Could you check a few things on this model? Use its own coordinates, in mm. Face numbers are marked on the shaded views. Round coordinates to 2 decimals unless told otherwise and drop trailing zeros. Loops run counter-clockwise (first coordinate to the right, second up) from the corner with the lowest first, then second, coordinate; pieces in that order, holes last. Notation, with made-up numbers: M 5.5,70.5 L 23.5,70.5 A13 cw 23.5,77.5 Z; hole C 68.5,58.25 d5. An arc over 180 degrees is marked long. Answer in a Markdown table with one row per item.
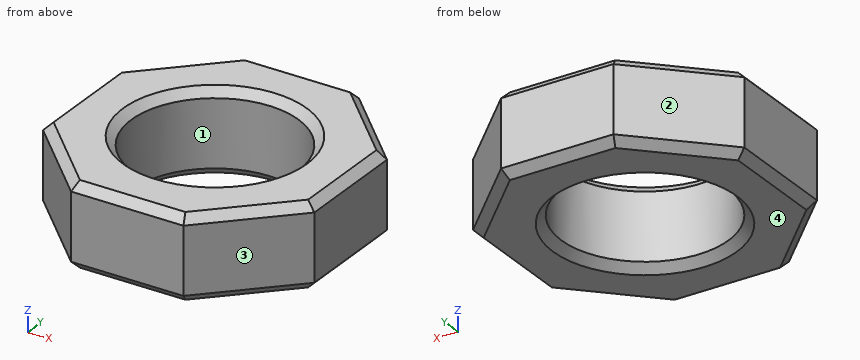
```python
from build123d import *

# Parameters (mm, degrees)
F1_DEPTH = 20
F2_R     = 20
F3_DEPTH = 20.001
F4_SIZE  = 2


with BuildPart() as f1:
    # F0 (on Top) → F1 (new body)
    with BuildSketch(Plane.XY):
        Polygon((32.5642426406, 13.3057863628), (13.6177850292, 32.4350085615), (-13.3057863628, 32.5642426406), (-32.4350085615, 13.6177850292), (-32.5642426406, -13.3057863628), (-13.6177850292, -32.4350085615), (13.3057863628, -32.5642426406), (32.4350085615, -13.6177850292), align=None)
    extrude(amount=F1_DEPTH)

    # F2 (on face) → F3 (cut, through all)
    with BuildSketch(Plane(origin=(0, 0, 0), x_dir=(1, 0, 0), z_dir=(0, 0, -1))):
        Circle(F2_R)
    extrude(amount=-F3_DEPTH, mode=Mode.SUBTRACT)

    # F4
    f4_edges = [f1.edges().sort_by_distance(p)[0] for p in [
        (23.091014, 22.870397, 20),
        (32.499626, -0.155999, 20),
        (0.155999, 32.499626, 20),
        (22.870397, -23.091014, 20),
        (-22.870397, 23.091014, 20),
        (-0.155999, -32.499626, 20),
        (-32.499626, 0.155999, 20),
        (-23.091014, -22.870397, 20),
        (-20, 0, 20),
        (23.091014, 22.870397, 0),
        (32.499626, -0.155999, 0),
        (0.155999, 32.499626, 0),
        (22.870397, -23.091014, 0),
        (-22.870397, 23.091014, 0),
        (-0.155999, -32.499626, 0),
        (-32.499626, 0.155999, 0),
        (-23.091014, -22.870397, 0),
        (-20, 0, 0),
    ]]
    chamfer(f4_edges, length=F4_SIZE)


solid = f1.part
```
1) I want a section at D-D, the plane y = 23. Please give me the cut outline in (x, z).
Computed:
| item | result |
|---|---|
| outline | M -22.96,2 L -20.12,0 L 20.15,0 L 22.96,2 L 22.96,18 L 20.15,20 L -20.12,20 L -22.96,18 Z |
2) Will these pins go through, and if not, where does the flat tip stop? P1, Ø2, axis at x = -1.5, z = 16.5, coming from the -Y side; P2, Ø1.5, axis at y = -24, z = 8, coming from the +X side; P3, Ø3, axis at x = 18, y = 2.5, coming from the -Z side; P4, Ø10, axis at x = -24.5, z = 12.5, coming from the -Y side.
Computed:
| item | result |
|---|---|
| P1 | stops at y = -32.5 |
| P2 | stops at x = 22.71 |
| P3 | passes through |
| P4 | stops at y = -26.5 |
3) I need wall thicknesses on line 1 (Y direction, x = -16, z = 10.25); line 2 (X direction, y = 0, z = 8.75); line 3 (X direction, y = -9, z = 13.5). Which ranges of each line are inside material? Lowest first, please.
Computed:
| item | result |
|---|---|
| line 1 | y = -30.03 to -12, 12 to 29.9 |
| line 2 | x = -32.5 to -20, 20 to 32.5 |
| line 3 | x = -32.54 to -17.86, 17.86 to 32.46 |
4) I want a section at B-B, the plane y = 0. Please give me the cut outline in (x, z), plus the area to 3 significant figures.
Computed:
| item | result |
|---|---|
| outline | M -32.5,2 L -30.5,0 L -22,0 L -20,2 L -20,18 L -22,20 L -30.5,20 L -32.5,18 Z; M 20,2 L 22,0 L 30.5,0 L 32.5,2 L 32.5,18 L 30.5,20 L 22,20 L 20,18 Z |
| area | 484 mm² |
5) If we mould it in two halves opening along Y, with no side actions, what happens to the marked faces 1, 2, 3 and 4? For each: released by +Y, released by -Y, zero draft, split by the parting line, or undercut.
Computed:
| item | result |
|---|---|
| face 1 | undercut |
| face 2 | released by +Y |
| face 3 | released by -Y |
| face 4 | zero draft |
6) I want a section at A-A, the plane z = 10.25. Please give me the cut outline in (x, y) (3 decimals).
Computed:
| item | result |
|---|---|
| outline | M -32.564,-13.306 L -13.618,-32.435 L 13.306,-32.564 L 32.435,-13.618 L 32.564,13.306 L 13.618,32.435 L -13.306,32.564 L -32.435,13.618 Z; hole C 0,0 d40 |
